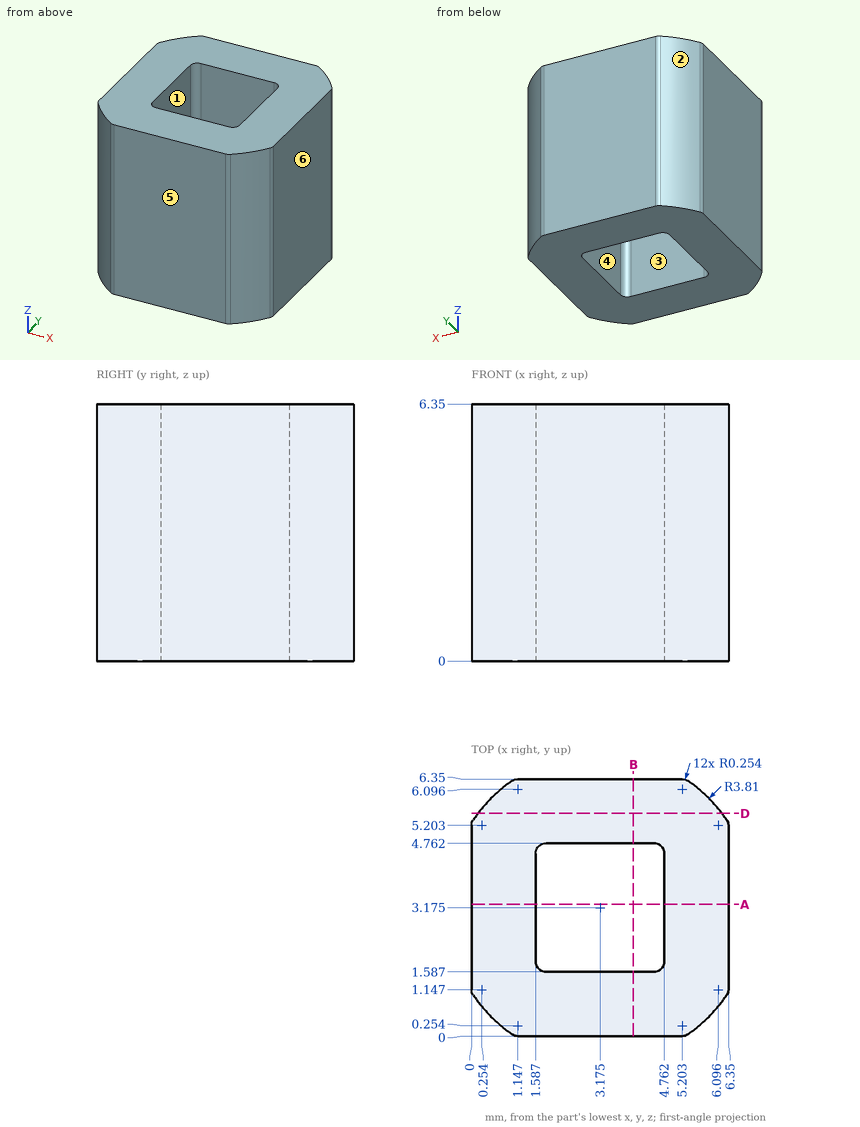
Geometry: see drawing. Coordinates: mm, zero at the bounding-box minimum. A direction names the side the tool comes from. Coordinates: 2 decimals unless noted, no trailing zeros. Write each loop counter-clockwise with the first axis right and the second up, starting at its lowest first coordinate (ties: lowest second). Pieces come first, ordered by that corner, then holes. Notation, with made-up numbers: (47.25, 17.25) - (69.25, 17.25) arc R33 ccw to (69.25, 50.25) - close; hole circle Ø2 at (40, -22.5). An arc over 180 degrees is marked (long way). Put each result on its own line as item: value. Start each with the question number.
1) Mould query, pull axis Y, two halves, no side actions, for the marked faces 3, 4, 5 and 6. Classes: pulls with the +Y half, pulls with the -Y half, needs draft (parallel to the pull), parting line crosses it, or undercut.
2) Ray query, L1, parallel to X at y = 2, z = 1.25; L2, parallel to Y at x = 5.25, z = 0.5 (1 decimal). Return the intervals inside material, ascending.
3) Reachability of the marked faces 1 and 2 from +Z, -Z, +X, -X, +Y, -Y: full face, straight path, thin tool, end or side. Return the list, or none.
4) Cut plane D-D (y = 5.5). Return the cut outline in (x, z).
5) Cut plane A-A (y = 3.25). Return the cut outline in (x, z).
Resolved:
1. face 3: undercut
1. face 4: undercut
1. face 5: pulls with the -Y half
1. face 6: needs draft
2. L1: x = 0 to 1.59, 4.76 to 6.35
2. L2: y = 0 to 6.3
3. face 1: +Z, -Z
3. face 2: +Z, -Z, -X, +Y
4. outline: (0.16, 0) - (6.19, 0) - (6.19, 6.35) - (0.16, 6.35) - close
5. outline: (0, 0) - (1.59, 0) - (1.59, 6.35) - (0, 6.35) - close; (4.76, 0) - (6.35, 0) - (6.35, 6.35) - (4.76, 6.35) - close
